```python
from build123d import *

# Parameters (mm, degrees)
F1_DEPTH = 19.05
F2_R     = 3.175
F3_DEPTH = 19.051
F5_DEPTH = 19.051


with BuildPart() as f1:
    # F0 (on Top) → F1 (new body)
    with BuildSketch(Plane.XY):
        with BuildLine():
            ThreePointArc((0, 6.35), (1.859872, 1.859872), (6.35, 0))
            Line((6.35, 0), (63.5, 0))
            ThreePointArc((63.5, 0), (67.990128, 1.859872), (69.85, 6.35))
            Line((69.85, 6.35), (69.85, 114.3))
            ThreePointArc((69.85, 114.3), (67.990128, 118.790128), (63.5, 120.65))
            Line((63.5, 120.65), (6.35, 120.65))
            ThreePointArc((6.35, 120.65), (1.859872, 118.790128), (0, 114.3))
            Line((0, 114.3), (0, 6.35))
        make_face()
    extrude(amount=F1_DEPTH)

    # F2 (on face) → F3 (cut, through all)
    with BuildSketch(Plane.XY.offset(19.05)):
        with Locations((34.925, 109.5375)):
            Circle(F2_R)
        with Locations((34.925, 11.1125)):
            Circle(F2_R)
        with BuildLine():
            Line((47.625, 98.425), (22.225, 98.425))
            ThreePointArc((22.225, 98.425), (13.244744, 94.705256), (9.525, 85.725))
            Line((9.525, 85.725), (9.525, 34.925))
            ThreePointArc((9.525, 34.925), (13.244744, 25.944744), (22.225, 22.225))
            Line((22.225, 22.225), (47.625, 22.225))
            ThreePointArc((47.625, 22.225), (56.605256, 25.944744), (60.325, 34.925))
            Line((60.325, 34.925), (60.325, 85.725))
            ThreePointArc((60.325, 85.725), (56.605256, 94.705256), (47.625, 98.425))
        make_face()
    extrude(amount=-F3_DEPTH, mode=Mode.SUBTRACT)

    # F4 (on face) → F5 (cut, through all)
    with BuildSketch(Plane.XY.offset(19.05)):
        with BuildLine():
            ThreePointArc((0, 62.452797), (0.489995, 63.186127), (1.355016, 63.014064))
            Line((1.355016, 63.014064), (9.292516, 55.076564))
            ThreePointArc((9.292516, 55.076564), (9.464579, 54.819052), (9.525, 54.515297))
            Line((9.525, 54.515297), (9.525, 85.725))
            ThreePointArc((9.525, 85.725), (13.244744, 94.705256), (22.225, 98.425))
            Line((22.225, 98.425), (47.625, 98.425))
            ThreePointArc((47.625, 98.425), (56.605256, 94.705256), (60.325, 85.725))
            Line((60.325, 85.725), (60.325, 62.452797))
            ThreePointArc((60.325, 62.452797), (60.814995, 63.186127), (61.680016, 63.014064))
            Line((61.680016, 63.014064), (69.617516, 55.076564))
            ThreePointArc((69.617516, 55.076564), (69.789579, 54.819052), (69.85, 54.515297))
            Line((69.85, 54.515297), (69.85, 114.3))
            ThreePointArc((69.85, 114.3), (67.990128, 118.790128), (63.5, 120.65))
            Line((63.5, 120.65), (6.35, 120.65))
            ThreePointArc((6.35, 120.65), (1.859872, 118.790128), (0, 114.3))
            Line((0, 114.3), (0, 62.452797))
        make_face()
    extrude(amount=-F5_DEPTH, mode=Mode.SUBTRACT)


solid = f1.part
```
CAD build for the part. Positions are in the model's coordinates, mm. A direction names the side the tool comes from. Round coordinates to 2 decimals unless told otherwise and drop trailing zeros. Order: outer loops, then holes, each group sorted by start corner. A loop starts at its lowest first (then second) coordinate and runs counter-clockwise, first axis right, second up. Notation, with made-up numbers: (-31.5, 4.25) - (-26.5, 4.25) arc R26 ccw to (-26.5, 29.25) - close; hole circle Ø4 at (87.5, 1.5). An arc over 180 degrees is marked (long way). Use CSV: the item, a comma, the result in double quotes. Start each with the question number.
1) Pin check, flat tip, straight feed: pin 1 Ø9.5 at (x, z) = (37.5, 6) entering from +Y (3 decimals). Stop position of the tip, or through.
2) Two-plate mould, pull along X, no slides. Class faces 1 (the cylindrical face through (1.81, 1.91, 9.39)), 2 (the flat face through (69.85, 30, 9)), 3 (the flat face through (34, 18, 0)), 4 (the flat face through (5.27, 59.1, 9.66)): pulls with the +X half, pulls with the -X half, needs draft (parallel to the pull), parting line crosses it, or undercut.
3) Saw through at D-D (x = 14). List the corners of the cut face in (y, z), and give its area (3 significant figures).
4) Saw through at A-A (y = 42.5). List the corners of the cut face in (x, z) (3 decimals).
5) Wall check: L1, parallel to X at y = 39, z = 14.5 (3 decimals); L2, parallel to Y at x = 25, z = 1 (3 decimals); L3, parallel to X at y = 13, z = 2.75. Give the ranges that are in metal, low to high. Write a range as [from, to].
6) Tool access for faces 5 (the flat face through (35, 22.225, 10)), 6 (the flat face through (65.593, 59.101, 9.658)): list every direction of +Z, -Z, +X, -X, +Y, -Y with a clear straight run to the whole face (end or side of a thin tool).
7) Saw through at B-B (x = 33.5). List the corners of the cut face in (y, z) (3 decimals), and give its area (3 significant figures).
Values follow:
1,pin 1,"stops at y = 22.225"
2,face 1,"pulls with the -X half"
2,face 2,"pulls with the +X half"
2,face 3,"needs draft"
2,face 4,"undercut"
3,outline,"(0, 0) - (25.25, 0) - (25.25, 19.05) - (0, 19.05) - close"
3,area,"481 mm2"
4,outline,"(0, 0) - (9.525, 0) - (9.525, 19.05) - (0, 19.05) - close; (60.325, 0) - (69.85, 0) - (69.85, 19.05) - (60.325, 19.05) - close"
5,L1,"x = [0, 9.525], [60.325, 69.85]"
5,L2,"y = [0, 22.225]"
5,L3,"x = [0, 32.37], [37.48, 69.85]"
6,face 5,"+Z, -Z, +Y"
6,face 6,"+Z, -Z, +X, +Y"
7,outline,"(0, 0) - (8.275, 0) - (8.275, 19.05) - (0, 19.05) - close; (13.95, 0) - (22.225, 0) - (22.225, 19.05) - (13.95, 19.05) - close"
7,area,"315 mm2"
